from build123d import *

# Parameters (mm, degrees)
BOX256_W          = 40
BOX256_H          = 20
BOX256_DEPTH      = 40
CYLINDER656_R     = 4.1
CYLINDER656_DEPTH = 10
CYLINDER657_R     = 11
CYLINDER657_DEPTH = 4
CHAMFER061_SIZE   = 2.5


with BuildPart() as krychle256:
    # Box256 → Box256 (new body)
    with BuildSketch(Plane(origin=(-20, 110, 30), x_dir=(1, 0, 0), z_dir=(0, 0, 1))):
        with Locations((20, 10)):
            Rectangle(BOX256_W, BOX256_H)
    extrude(amount=BOX256_DEPTH)


with BuildPart() as obj1:
    # Cylinder656 → Cylinder656 (new body)
    with BuildSketch(Plane(origin=(0, 118, 50), x_dir=(1, 0, 0), z_dir=(0, -1, 0))):
        Circle(CYLINDER656_R)
    extrude(amount=CYLINDER656_DEPTH)


with BuildPart() as chamfer061:
    # Cylinder657 → Cylinder657 (new body)
    with BuildSketch(Plane(origin=(0, 110, 50), x_dir=(1, 0, 0), z_dir=(0, -1, 0))):
        Circle(CYLINDER657_R)
    extrude(amount=CYLINDER657_DEPTH)

    # Cut265: cut obj1
    add(obj1.part, mode=Mode.SUBTRACT)

    # Cut552: cut Krychle256
    add(krychle256.part, mode=Mode.SUBTRACT)

    # Chamfer061
    chamfer061_edges = [chamfer061.edges().sort_by_distance(p)[0] for p in [
        (-11, 110, 50),
    ]]
    chamfer(chamfer061_edges, length=CHAMFER061_SIZE)


solid = chamfer061.part
Check sheet for the modelled part. Datum: model origin and axes. Units: mm. Round coordinates to 2 decimals unless told otherwise and drop trailing zeros. Order: outer loops, then holes, each group sorted by start corner. A loop starts at its lowest first (then second) coordinate and runs counter-clockwise, first axis right, second up.
(1) Draft check along Z on faces 1 (the flat face through (0, 106, 50)), 2 (the cylindrical face through (-3.022, 109.014, 52.771)), 3 (the cylindrical face through (-8.11, 106.76, 57.43)), 4 (the flat face through (0, 108, 50)). Enter one of: pulls with the +Z half, pulls with the -Z half, needs draft (parallel to the pull), parting line crosses it, or undercut.
(2) Scan lines: probe 1 along Z at (x, y) = (6.5, 107.8); probe 2 along X at (y, z) = (108.1, 49.75); probe 3 along Z at (x, y) = (-3.5, 109.6). Record each from-to range of solid material in increasing order.
(3) Cross-section at D-D, the plane y = 106.75. Enter the section's corners in (x, z).
(4) Cross-section at B-B, the plane x = 0. Enter the section's corners in (y, z), and give its area (4 significant figures).
(5) Cross-section at C-C, the plane y = 108.9. Enter the section's corners in (x, z).
(6) Cross-section at A-A, the plane z = 50. Enter the section's corners in (x, y), and give its area (4 significant figures).
Check sheet entries:
1. face 1: needs draft
1. face 2: undercut
1. face 3: parting line crosses it
1. face 4: undercut
2. probe 1: z = 41.5 to 58.5
2. probe 2: x = -10.4 to -4.09, 4.09 to 10.4
2. probe 3: z = 41.82 to 47.86, 52.14 to 58.18
3. outline: circle Ø22 at (0, 50)
4. outline: (106, 39) - (107.5, 39) - (110, 41.5) - (110, 45.9) - (108, 45.9) - (108, 54.1) - (110, 54.1) - (110, 58.5) - (107.5, 61) - (106, 61) - close
4. area: 65.35 mm2
5. outline: circle Ø19.2 at (0, 50); hole circle Ø8.2 at (0, 50)
6. outline: (-11, 106) - (11, 106) - (11, 107.5) - (8.5, 110) - (4.1, 110) - (4.1, 108) - (-4.1, 108) - (-4.1, 110) - (-8.5, 110) - (-11, 107.5) - close
6. area: 65.35 mm2
